from build123d import *
from build123d.topology import SkipClean

# Parameters (mm, degrees)
BASE_FLANGE1_DEPTH                           = 13.5
CBORE_FOR_M8_HEX_SOCKET_HEAD_CAP_SCR_2_COUNT = 2
CBORE_FOR_M8_HEX_SOCKET_HEAD_CAP_SCR_2_PITCH = 30
M4_TAPPED_HOLE1_AT_2_COUNT                   = 2
M4_TAPPED_HOLE1_AT_2_PITCH                   = 29.69848481
M4_TAPPED_HOLE1_AT_3_COUNT                   = 2
M4_TAPPED_HOLE1_AT_3_PITCH                   = 42
M4_TAPPED_HOLE1_AT_4_COUNT                   = 2
M4_TAPPED_HOLE1_AT_4_PITCH                   = 29.69848481
CIRPATTERN1_COUNT                            = 4
FILLET2_R                                    = 6
FILLET1_R                                    = 2
CHAMFER1_SIZE                                = 0.8


# Sheet-metal steps are written as plain solids
with BuildPart() as part:
    # Sketch1 → Base-Flange1 (new body)
    with BuildSketch(Plane.XY):
        with BuildLine():
            Line((0, 0), (-65, 0))
            Line((-65, 0), (-65, 60))
            Line((-65, 60), (-32.5, 78.763883749))
            Line((-32.5, 78.763883749), (-32.5, 102.5))
            Line((-32.5, 102.5), (0, 102.5))
            Line((0, 102.5), (0, 87))
            ThreePointArc((0, 87), (-17, 70), (0, 53))
            Line((0, 53), (0, 0))
        make_face()
    extrude(amount=-BASE_FLANGE1_DEPTH)

    # Sketch7 → CBORE for M8 Hex Socket Head Cap Screw1 (revolve, cut)
    with BuildSketch(Plane(origin=(-50, 45, -13.5), x_dir=(0, 1, 0), z_dir=(1, 0, 0))):
        Polygon((0, 0), (0, 13.5), (4.525, 13.5), (4.25, 13.225), (4.25, 8.6), (7, 8.6), (7, 0.525), (7.525, 0), align=None)
    cbore_for_m8_hex_socket_head_cap_screw1 = revolve(axis=Axis((-50, 45, -19.85), (0, 0, 1)), mode=Mode.SUBTRACT)

    # CBORE for M8 Hex Socket Head Cap Scr 2: CBORE for M8 Hex Socket Head Cap Screw1 ×2
    with Locations(*[(0, -i * CBORE_FOR_M8_HEX_SOCKET_HEAD_CAP_SCR_2_PITCH, 0) for i in range(1, CBORE_FOR_M8_HEX_SOCKET_HEAD_CAP_SCR_2_COUNT)]):
        add(cbore_for_m8_hex_socket_head_cap_screw1, mode=Mode.SUBTRACT)

    # Sketch17 → CBORE for M6 Hex Socket Head Cap Screw1 (revolve, cut)
    with BuildSketch(Plane(origin=(-20, 15, -13.5), x_dir=(0, 1, 0), z_dir=(1, 0, 0))):
        Polygon((0, 0), (0, 13.5), (3.5, 13.5), (3.25, 13.25), (3.25, 6.5), (5.5, 6.5), (5.5, 0.25), (5.75, 0), align=None)
    revolve(axis=Axis((-20, 15, -19.85), (0, 0, 1)), mode=Mode.SUBTRACT)

    # Mirror1: part across plane


with BuildPart() as part_1:
    with SkipClean():  # the faces are left unmerged after this step: merging them gives an invalid solid
        add(part.part)
        add(part.part.mirror(Plane(origin=(0, 102.5, -13.5), x_dir=(0, 0, 1), z_dir=(1, 0, 0))))

    # Sketch12 → M4 Tapped Hole1 (revolve, cut)
    with SkipClean():  # the faces are left unmerged after this step: merging them gives an invalid solid
        with BuildSketch(Plane(origin=(-21, 70, 0), x_dir=(0, -1, 0), z_dir=(1, 0, 0))):
            Polygon((0, 0), (0, 13.5), (2, 13.5), (1.65, 13.15), (1.65, 0.35), (2, 0), align=None)
        m4_tapped_hole1 = revolve(axis=Axis((-21, 70, 6.35), (0, 0, -1)), mode=Mode.SUBTRACT)

    # M4 Tapped Hole1 at 2: M4 Tapped Hole1 ×2
    with SkipClean():  # the faces are left unmerged after this step: merging them gives an invalid solid
        with Locations(*[Vector(0.7071067811865477, 0.7071067811865474, 0) * (i * M4_TAPPED_HOLE1_AT_2_PITCH) for i in range(1, M4_TAPPED_HOLE1_AT_2_COUNT)]):
            add(m4_tapped_hole1, mode=Mode.SUBTRACT)

    # M4 Tapped Hole1 at 3: M4 Tapped Hole1 ×2
    with SkipClean():  # the faces are left unmerged after this step: merging them gives an invalid solid
        with Locations(*[(i * M4_TAPPED_HOLE1_AT_3_PITCH, 0, 0) for i in range(1, M4_TAPPED_HOLE1_AT_3_COUNT)]):
            add(m4_tapped_hole1, mode=Mode.SUBTRACT)

    # M4 Tapped Hole1 at 4: M4 Tapped Hole1 ×2
    with SkipClean():  # the faces are left unmerged after this step: merging them gives an invalid solid
        with Locations(*[Vector(0.7071067811865476, -0.7071067811865475, 0) * (i * M4_TAPPED_HOLE1_AT_4_PITCH) for i in range(1, M4_TAPPED_HOLE1_AT_4_COUNT)]):
            add(m4_tapped_hole1, mode=Mode.SUBTRACT)

    # Sketch15 → M4 Tapped Hole2 (revolve, cut)
    with SkipClean():  # the faces are left unmerged after this step: merging them gives an invalid solid
        with BuildSketch(Plane(origin=(23.550191347, 93.550191347, -13.5), x_dir=(0, 1, 0), z_dir=(1, 0, 0))):
            Polygon((0, 0), (0, 13.5), (2.275, 13.5), (1.65, 12.875), (1.65, 0.625), (2.275, 0), align=None)
        m4_tapped_hole2 = revolve(axis=Axis((23.550191347, 93.550191347, -19.85), (0, 0, 1)), mode=Mode.SUBTRACT)

    # CirPattern1: M4 Tapped Hole2 ×4 about axis
    with SkipClean():  # the faces are left unmerged after this step: merging them gives an invalid solid
        cirpattern1_axis = Axis((0, 70, 0), (0, 0, 1))
        for i in range(1, CIRPATTERN1_COUNT):
            add(m4_tapped_hole2.rotate(cirpattern1_axis, i * 360 / CIRPATTERN1_COUNT), mode=Mode.SUBTRACT)

    # Fillet2
    fillet2_edges = [part_1.edges().sort_by_distance(p)[0] for p in [
        (-32.5, 78.763883749, -6.75),
        (32.5, 78.763883749, -6.75),
    ]]
    fillet(fillet2_edges, radius=FILLET2_R)

    # Fillet1
    fillet1_edges = [part_1.edges().sort_by_distance(p)[0] for p in [
        (-65, 60, -6.75),
        (-32.5, 102.5, -6.75),
        (-65, 0, -6.75),
        (65, 60, -6.75),
        (32.5, 102.5, -6.75),
        (65, 0, -6.75),
    ]]
    fillet(fillet1_edges, radius=FILLET1_R)

    # Chamfer1
    chamfer1_edges = [part_1.edges().sort_by_distance(p)[0] for p in [
        (-17, 70, 0),
        (-17, 70, -13.5),
        (49.75, 68.804591605, 0),
        (49.75, 68.804591605, -13.5),
        (-49.75, 68.804591605, 0),
        (-49.75, 68.804591605, -13.5),
        (33.303847577, 79.227985364, 0),
        (33.303847577, 79.227985364, -13.5),
        (-33.303847577, 79.227985364, 0),
        (-33.303847577, 79.227985364, -13.5),
        (65, 30.422649731, 0),
        (65, 30.422649731, -13.5),
        (32.5, 91.363992682, 0),
        (-15.25, 102.5, 0),
        (-32.5, 91.363992682, 0),
        (-65, 30.422649731, 0),
        (-31.5, 0, 0),
        (-64.414213562, 0.585786438, 0),
        (64.414213562, 0.585786438, 0),
        (-31.914213562, 101.914213562, 0),
        (31.914213562, 101.914213562, 0),
        (-64.732050808, 59.845299462, 0),
        (64.732050808, 59.845299462, 0),
        (-15.25, 102.5, -13.5),
        (32.5, 91.363992682, -13.5),
        (-31.5, 0, -13.5),
        (-65, 30.422649731, -13.5),
        (-32.5, 91.363992682, -13.5),
        (-64.414213562, 0.585786438, -13.5),
        (64.414213562, 0.585786438, -13.5),
        (-31.914213562, 101.914213562, -13.5),
        (31.914213562, 101.914213562, -13.5),
        (-64.732050808, 59.845299462, -13.5),
        (64.732050808, 59.845299462, -13.5),
    ]]
    chamfer(chamfer1_edges, length=CHAMFER1_SIZE)


solid = part_1.part
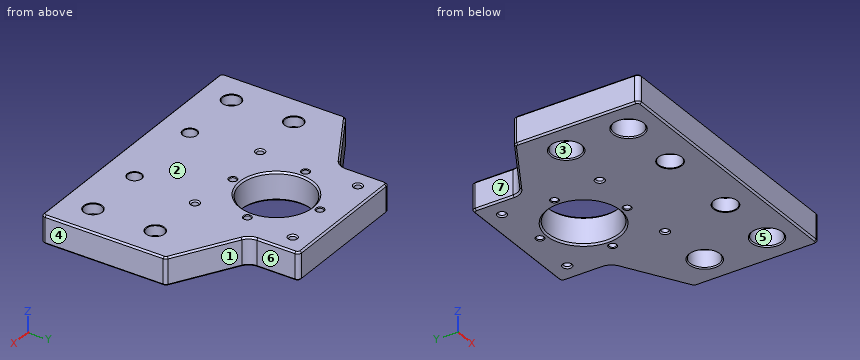
CAD build for the part. Positions are in the model's coordinates, mm. Face numbers are marked on the shaded views. A direction names the side the tool comes from. Give positions to 0.01 mm unless a question says otherwise; leave off trailing zeros. Answer in a Markdown table with one row per item.
1. Saw through at A-A, the plane x = 50. Count the separate pieces of the cut face and the enclosed holes in it, plus the area to 3 significant figures.
Data:
| item | result |
|---|---|
| separate pieces | 3 |
| enclosed holes | 0 |
| area | 601 mm² |
2. Flat gauge pins, fed straight in: pin 1 (9 mm diameter, centred on x = -21, y = 14.5, fed in from -Z); pin 2 (7 mm diameter, centred on x = 53, y = 14.5, fed in from -Z); pin 3 (5 mm diameter, centred on y = 89.5, z = -2.5, fed in from +X). Where does each tip first touch, or does it go through?
Data:
| item | result |
|---|---|
| pin 1 | stops at z = -13.37 |
| pin 2 | stops at z = -4.9 |
| pin 3 | stops at x = 32.5 |
3. Tool access for the marked faces 4, 5, 6 and 7: list every direction of +Z, -Z, +X, -X, +Y, -Y with a clear straight run to the whole face (end or side of a thin tool).
Data:
| item | result |
|---|---|
| face 4 | +Z, -Z, +X, +Y, -Y |
| face 5 | -Z |
| face 6 | +Z, -Z, +X, +Y |
| face 7 | +Z, -Z, -X, +Y |
4. Pull direction X, two halves, no side cores. Call the marked faces 1, 2 and 3: pulls with the +X half, pulls with the -X half, needs draft (parallel to the pull), parting line crosses it, or undercut.
Data:
| item | result |
|---|---|
| face 1 | pulls with the +X half |
| face 2 | needs draft |
| face 3 | undercut |
5. Probe probe 1 along X at (y, z) = (15, -1.6); probe 2 along X at (y, z) = (15, -9.75); probe 3 along Y at (x, z) = (51.5, -5). List the from-to ranges inside material, lowest first. Write a range as [from, to].
Data:
| item | result |
|---|---|
| probe 1 | x = [-65, -54.25], [-45.75, -23.25], [-16.75, 16.75], [23.25, 45.75], [54.25, 65] |
| probe 2 | x = [-65, -57], [-43, -25.5], [-14.5, 14.5], [25.5, 43], [57, 65] |
| probe 3 | y = [0, 8.16], [21.84, 38.16], [51.84, 67.79] |
